Job drawing, mm, ordinate dimensions from the low corner. One solid piece. Give positions to 0.01 mm unless a question says otherwise; leave off trailing zeros. Loops run counter-clockwise (first coordinate to the right, second up) from the corner with the lowest first, then second, coordinate; pieces in that order, holes last. Notation, with made-up numbers: (-21.75, 75.5) - (28.25, 75.5) arc R27 cw to (28.25, 114.5) - close; hole circle Ø3 at (57, -27.5). An arc over 180 degrees is marked (long way). Answer as CSV lines item,"result". Start each with the question number.
Item 1: Saw through at D-D on x = 7.5. Give the cut face in (y, z), plus the area to 3 significant figures.
Item 2: Drill centre lines: L1, parallel to Z at x = 17.5, y = 1.25; L2, parallel to Z at x = 16.5, y = 1.9; L3, parallel to Z at x = 11.5, y = 1.35. Where is each one in solid material? Low to high. Write a range as from..to.
Item 3: Saw through at B-B on y = 1.3. Give the cut face in (x, z), plus the area to 3 significant figures.
Item 4: Pin check, flat tip, straight feed: pin 1 (4 mm diameter, centred on x = 17.5, z = 17.5, fed in from -Y). Stop position of the tip, or through.
Item 5: Saw through at C-C on z = 28. Give the cut face in (x, y).
Item 6: Saw through at A-A on z = 17.5. Give the cut face in (x, y).
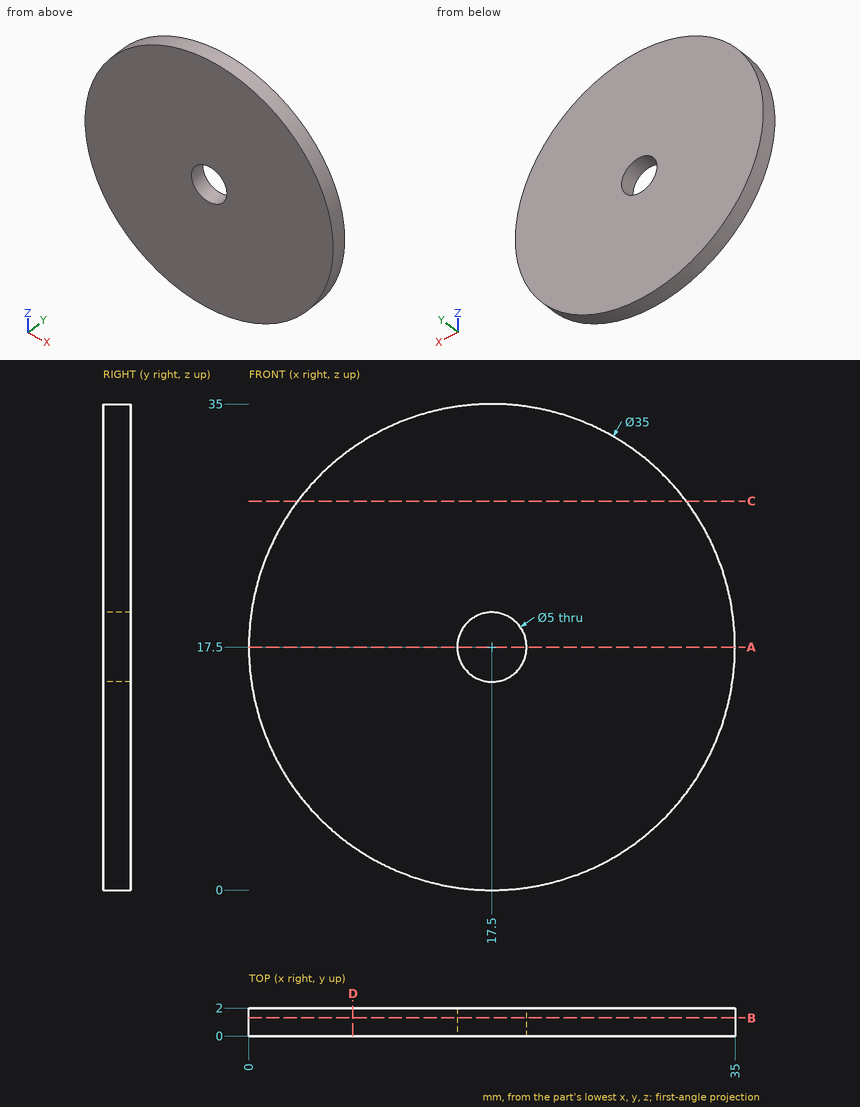
Responses:
1,outline,"(0, 3.14) - (2, 3.14) - (2, 31.86) - (0, 31.86) - close"
1,area,"57.4 mm2"
2,L1,"0..15, 20..35"
2,L2,"0.03..15.21, 19.79..34.97"
2,L3,"1.06..33.94"
3,outline,"circle Ø35 at (17.5, 17.5); hole circle Ø5 at (17.5, 17.5)"
3,area,"942 mm2"
4,pin 1,"through"
5,outline,"(3.5, 0) - (31.5, 0) - (31.5, 2) - (3.5, 2) - close"
6,outline,"(0, 0) - (15, 0) - (15, 2) - (0, 2) - close; (20, 0) - (35, 0) - (35, 2) - (20, 2) - close"
